```python
from build123d import *

# Parameters (mm, degrees)
F1_DEPTH = 100
F3_DEPTH = 100
F4_W     = 44.336
F4_H     = 25
F4_W_2   = 45.646268
F4_H_2   = 27.82878
F4_W_3   = 44.991
F5_DEPTH = 114
F7_DEPTH = 25


with BuildPart() as f1:
    # F0 (on Front) → F1 (new body)
    with BuildSketch(Plane.XZ):
        Polygon((0, 90), (0, 0), (148.54021, 0), (148.54021, 110.875965), align=None)
    extrude(amount=F1_DEPTH)

    # F2 (on face) → F3 (cut)
    with BuildSketch(Plane.XZ.offset(100)):
        Polygon((108.54021, 0), (141.54021, 0), (141.54021, 70), (108.54021, 105.254332), (0, 90), (0, 0), align=None)
    extrude(amount=-F3_DEPTH, mode=Mode.SUBTRACT)

    # F4 (on face) → F5 (cut)
    with BuildSketch(Plane(origin=(0, 0, 0), x_dir=(1, 0, 0), z_dir=(0, 0, -1))):
        with Locations((119.37221, 77.5)):
            Rectangle(F4_W, F4_H)
        with Locations((118.717076, 6.08561)):
            Rectangle(F4_W_2, F4_H_2)
        with Locations((119.04471, 42.5)):
            Rectangle(F4_W_3, F4_H)
    extrude(amount=-F5_DEPTH, mode=Mode.SUBTRACT)

    # F6 (on face) → F7 (cut)
    with BuildSketch(Plane(origin=(141.54021, 0, 0), x_dir=(0, -1, 0), z_dir=(-1, 0, 0))):
        with BuildLine():
            ThreePointArc((52.5, 35), (70, 17.5), (87.5, 35))
            Line((87.5, 35), (52.5, 35))
        make_face()
        with BuildLine():
            Line((52.5, 35), (87.5, 35))
            ThreePointArc((87.5, 35), (70, 52.5), (52.5, 35))
        make_face()
    extrude(amount=-F7_DEPTH, mode=Mode.SUBTRACT)


solid = f1.part
```
CAD build for the part. Positions are in the model's coordinates, mm. A direction names the side the tool comes from. Coordinates: 2 decimals unless noted, no trailing zeros. Loops run counter-clockwise (first coordinate to the right, second up) from the corner with the lowest first, then second, coordinate; pieces in that order, holes last. Notation, with made-up numbers: (48.5, 19) - (60.5, 19) arc R12 ccw to (60.5, 25) - close; hole circle Ø11 at (34.5, -39). An arc over 180 degrees is marked (long way). Return JSON: item names as keys, results as strings.
1. Band-saw the part on C-C (x = 128). Give the cut face in (y, z).
Result:
{"outline": "(-100, 84.47) - (-90, 84.47) - (-90, 107.99) - (-100, 107.99) - close; (-65, 84.47) - (-55, 84.47) - (-55, 107.99) - (-65, 107.99) - close; (-30, 84.47) - (-20, 84.47) - (-20, 107.99) - (-30, 107.99) - close"}
2. Band-saw the part on D-D (y = -22). Give the cut face in (x, z), and give its area (3 significant figures).
Result:
{"outline": "(108.54, 105.25) - (141.54, 70) - (141.54, 0) - (148.54, 0) - (148.54, 110.88) - close", "area": "1,430 mm2"}
3. Band-saw the part on B-B (y = -70). Give the cut face in (x, z), and give its area (3 significant figures).
Result:
{"outline": "(141.54, 0) - (148.54, 0) - (148.54, 17.5) - (141.54, 17.5) - close; (141.54, 52.5) - (148.54, 52.5) - (148.54, 110.88) - (141.54, 109.89) - close", "area": "528 mm2"}
4. 3-axis set-ups, long thin cutter, end or side, ignore diameter. For faces 4 (the flat face through (132, -90, 94)), 5 (the flat face through (145, 0, 56)), 6 (the flat face through (141.54, -49, 54)): which of +Z, -Z, +X, -X, +Y, -Y reach the whole face in a straight line?
Result:
{"face 4": "+Z, -Z, -X", "face 5": "+Z, -Z, +X, -X, +Y", "face 6": "-Z, -X"}
5. Probe L1, parallel to Y at x = 133, z = 90; L2, parallel to X at y = -18, z = 98; L3, parallel to Z at x = 144.75, y = -70. List the from-to ranges inside material, lowest first. Write a range as from..to.
Result:
{"L1": "y = -100..-90, -65..-55, -30..-20", "L2": "x = 141.54..148.54", "L3": "z = 0..17.5, 52.5..110.34"}
6. Mould opens along Y. For faces 1 (the flat face through (145, -49, 0)), 2 (the flat face through (132, -30, 94)), 3 (the flat face through (132, -20, 94)) say: released by +Y, released by -Y, zero draft, split by the parting line, or undercut.
Result:
{"face 1": "zero draft", "face 2": "undercut", "face 3": "released by +Y"}
7. Band-saw the part on A-A (z = 35). Give the cut face in (x, y).
Result:
{"outline": "(141.54, -100) - (148.54, -100) - (148.54, -87.5) - (141.54, -87.5) - close; (141.54, -52.5) - (148.54, -52.5) - (148.54, 0) - (141.54, 0) - close"}
8. Drop flat-ended pins along their axis: pin 1 (1 mm diameter, centred on x = 128, y = -23, fed in from +Z); pin 2 (12 mm diameter, centred on x = 114, y = -75, fed in from +Z); pin 3 (6 mm diameter, centred on x = 140, y = -45.5, fed in from +Z); pin 4 (4 mm diameter, centred on x = 143, y = -11.5, fed in from +Z). Give the stop position or say it passes through.
Result:
{"pin 1": "stops at z = 108.06", "pin 2": "passes through", "pin 3": "stops at z = 110.1", "pin 4": "stops at z = 110.38"}
